Can you work these out from the model? Positions are in its coordinate system, mm. Face numbers are marked on the shaded views. A direction names the side the tool comes from. Round coordinates to 2 decimals unless told otherwise and drop trailing zeros. Write each loop counter-clockwise with the first axis right and the second up, starting at its lowest first coordinate (ties: lowest second). Pieces come first, ordered by that corner, then holes. Notation, with made-up numbers: M 33.5,66.5 L 78.5,66.5 A23 cw 78.5,76.5 Z; hole C 47,12 d5. An arc over 180 degrees is marked long. Answer as a JSON object with one key per item and string values. Group by question number.
1) Suppose I cut it at D-D, the plane z = 34. Write out the boundary of the cut face in (x, y), and give its area (3 significant figures).
2) I'm going to push flat-ended pins straight in: pin 1 Ø8 at (x, y) = (67.5, -98) entering from -Z; pin 2 Ø12 at (y, z) = (-55.5, 67.5) entering from +X; pin 3 Ø19 at (x, y) = (47.5, -100) entering from +Z; pin 4 Ø6 at (x, z) = (-83, 5.5) entering from +Y. Where does each tip first touch, or does it pass through?
3) Suppose I cut it at C-C, the plane x = 42. Write out the boundary of the cut face in (y, z), and give its area (3 significant figures).
4) If we mould it in two halves opening along Y, with no side actions, what happens to the marked faces 4, 5 and 6? For each: +Y half, -Y half, draft (parallel to the pull), parting line (faces both ways), or undercut.
5) Suppose I cut it at A-A, the plane z = 74. Write out the boundary of the cut face in (x, y).
6) On a 3-axis mill with a long thin cutter (end or side, diameter ignored), from which of +Z, -Z, +X, -X, +Y, -Y can I reach the whole of each face in a straight line? I mean the marked faces 1, 2 and 3. Say none if no direction works.
7) Please list where these lines run through material, in increasing order: L1, parallel to X at y = -53.5, z = 82; L2, parallel to Y at x = -102, z = 5; L3, parallel to Z at x = 27, y = -56.5. Write a range as [from, to].
8) Suppose I cut it at B-B, the plane x = -99. Write out the boundary of the cut face in (y, z).
from build123d import *

# Parameters (mm, degrees)
F1_DEPTH  = 25
F3_DEPTH  = 13
F4_W      = 76
F4_H      = 26
F5_DEPTH  = 89
F7_DEPTH  = 26.001
F9_R      = 19
F10_DEPTH = 26.001
F9_R_2    = 28.5
F11_DEPTH = 1
F12_R     = 6


with BuildPart() as f1:
    # F0 (on Right) → F1 (new body)
    with BuildSketch(Plane.YZ):
        Polygon((-127, 0), (0, 0), (0, 50), (-89, 139), (-127, 139), align=None)
    extrude(amount=F1_DEPTH)

    # F2 (on face) → F3 (join)
    with BuildSketch(Plane(origin=(0, 0, 0), x_dir=(0, -1, 0), z_dir=(-1, 0, 0))):
        Polygon((0, 24), (0, 0), (127, 0), (127, 139), (115, 139), align=None)
    extrude(amount=F3_DEPTH)

    # F4 (on face) → F5 (join)
    with BuildSketch(Plane.YZ.offset(25)):
        with Locations((-89, 13)):
            Rectangle(F4_W, F4_H)
    extrude(amount=F5_DEPTH)

    # F6 (on face) → F7 (cut, through all)
    with BuildSketch(Plane.XY.offset(26)):
        with BuildLine():
            ThreePointArc((76, -51), (102.8700576851, -62.1299423149), (114, -89))
            Line((114, -89), (114, -51))
            Line((114, -51), (76, -51))
        make_face()
        with BuildLine():
            Line((114, -127), (114, -89))
            ThreePointArc((114, -89), (102.8700576851, -115.8700576851), (76, -127))
            Line((76, -127), (114, -127))
        make_face()
    extrude(amount=-F7_DEPTH, mode=Mode.SUBTRACT)

    # F9 (on face) → F10 (cut, through all)
    with BuildSketch(Plane.XY.offset(26)):
        with Locations((76, -89)):
            Circle(F9_R)
    extrude(amount=-F10_DEPTH, mode=Mode.SUBTRACT)

    # F9 (on face) → F11 (cut)
    with BuildSketch(Plane.XY.offset(26)):
        with Locations((76, -89)):
            Circle(F9_R_2)
        with Locations((76, -89)):
            Circle(F9_R, mode=Mode.SUBTRACT)
    extrude(amount=-F11_DEPTH, mode=Mode.SUBTRACT)

    # F12
    f12_edges = [f1.edges().sort_by_distance(p)[0] for p in [
        (50.5, -51, 26),
        (50.5, -127, 26),
        (114, -89, 26),
    ]]
    fillet(f12_edges, radius=F12_R)

    # F13: F1 across plane


with BuildPart() as f1_1:
    add(f1.part)
    add(f1.part.mirror(Plane.YZ.offset(-13)))


solid = f1_1.part
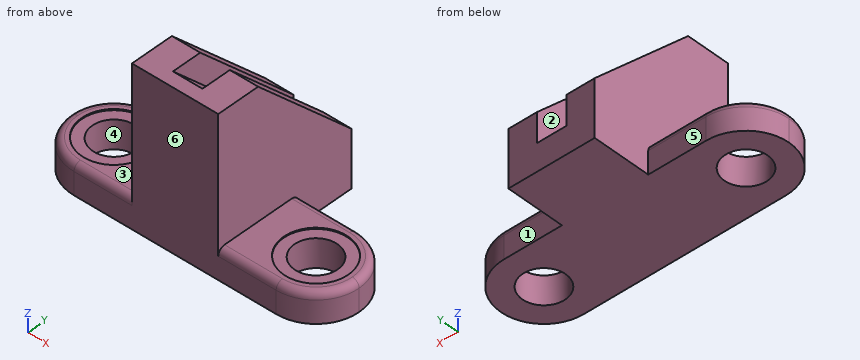
Results:
{
 "1": {"outline": "M -51,-127 L 25,-127 L 25,0 L 0,0 L 0,-10 L -26,-10 L -26,0 L -51,0 Z", "area": "9,390 mm^2"},
 "2": {"pin 1": "through", "pin 2": "x = 25", "pin 3": "z = 26", "pin 4": "y = -51"},
 "3": {"outline": "M -127,0 L -51,0 L -51,20 A6 ccw -57,26 L -121,26 A6 ccw -127,20 Z", "area": "1,960 mm^2"},
 "4": {"face 4": "undercut", "face 5": "+Y half", "face 6": "-Y half"},
 "5": {"outline": "M -51,-127 L 25,-127 L 25,-24 L 0,-24 L 0,-50 L -26,-50 L -26,-24 L -51,-24 Z"},
 "6": {"face 1": "+Z, -Z, +X, +Y", "face 2": "+Z, +Y", "face 3": "+Z, -X, +Y, -Y"},
 "7": {"L1": "[-51, -26], [0, 25]", "L2": "[-127, -108], [-70, -51]", "L3": "[0, 25.98]"},
 "8": {"outline": "M -127,0 L -107.76,0 L -107.76,25 L -117.34,25 L -117.34,26 L -121,26 A6 ccw -127,20 Z; M -70.24,0 L -51,0 L -51,20 A6 ccw -57,26 L -60.66,26 L -60.66,25 L -70.24,25 Z"}
}
